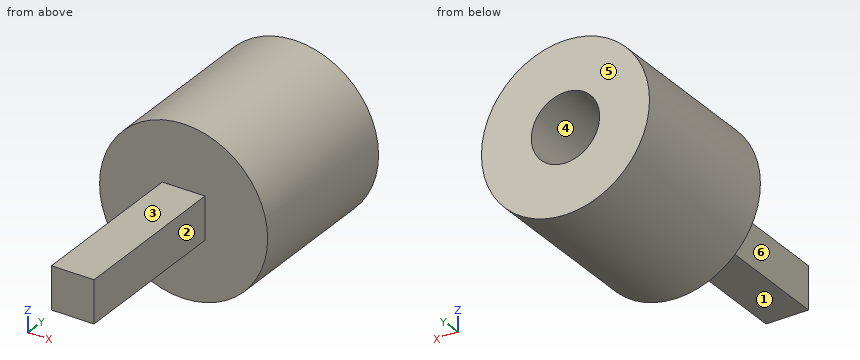
Autodesk Inventor part; units mm, degrees
ref_plane "YZ Plane" through (0, 0, 0) normal (1, 0, 0) x (0, 1, 0)
ref_plane "XZ Plane" through (0, 0, 0) normal (0, 1, 0) x (-1, 0, 0)
ref_plane "XY Plane" through (0, 0, 0) normal (0, 0, 1) x (1, 0, 0)
sketch "草圖1" plane through (0, 0, 0) normal (0, 1, 0) x (-1, 0, 0)
  circle A0 centre (0, 0) radius 7.5
  dimension "d0" = 15
extrude "擠出1" add sketch "草圖1" along normal blind 15
sketch "草圖2" plane through (0, 15, 0) normal (0, 1, 0) x (1, 0, 0)
  circle A0 centre (0, 0) radius 3.05
  dimension "d3" = 6.1
extrude "擠出2" cut sketch "草圖2" against normal blind 12
sketch "草圖3" plane through (0, 0, 0) normal (0, -1, 0) x (1, 0, 0)
  line L0 (1.9, 1.9) -> (-1.9, 1.9)
  line L1 (-1.9, 1.9) -> (-1.9, -1.9)
  line L2 (-1.9, -1.9) -> (1.9, -1.9)
  line L3 (1.9, -1.9) -> (1.9, 1.9)
  circle A0 centre (0, 0) radius 3.05
  line L4 (1.9, 1.9) -> (-1.9, -1.9) construction
  line L5 (-1.9, 1.9) -> (1.9, -1.9) construction
  dimension "d6" = 3.8
  dimension "d7" = 3.8
extrude "擠出3" add sketch "草圖3" along normal blind 15 contours L3 L2 L1 L0
properties part number "transfer"
The model under review builds one solid part; all positions refer to its coordinate system, in mm. Face numbers are marked on the shaded views. A direction names the side the tool comes from. Round coordinates to 2 decimals unless told otherwise and drop trailing zeros. Write each loop counter-clockwise with the first axis right and the second up, starting at its lowest first coordinate (ties: lowest second). Pieces come first, ordered by that corner, then holes. Notation, with made-up numbers: (73, 25) -> (95, 25) arc R11 cw to (95, 29) -> close; hole circle Ø11 at (22.5, 53.25). An arc over 180 degrees is marked (long way). Use CSV: the item, a comma, the result in double quotes.
Q1. To check wall thickness, follow probe 1 along Z at (x, y) = (0, 9); probe 2 along Y at (x, z) = (-3.75, -4.25); probe 3 along Z at (x, y) = (0.25, -5.5). State the ranges of each line that lie inside material, in increasing order. Write a range as [from, to].
Checks:
probe 1,"[-7.5, -3.05], [3.05, 7.5]"
probe 2,"[0, 15]"
probe 3,"[-1.9, 1.9]"
Q2. Consider section D-D (y = 10.25). Give the boundary of the cut face in (x, z).
Checks:
outline,"circle Ø15 at (0, 0); hole circle Ø6.1 at (0, 0)"
Q3. Mouldability with a two-part tool opening along X and no side actions: class the marked faces 4, 5 and 6 as released by +X, released by -X, zero draft, split by the parting line, or undercut.
Checks:
face 4,"undercut"
face 5,"zero draft"
face 6,"released by -X"
Q4. Consider section C-C (y = -11.5). Give the boundary of the cut face in (x, z).
Checks:
outline,"(-1.9, -1.9) -> (1.9, -1.9) -> (1.9, 1.9) -> (-1.9, 1.9) -> close"
Q5. Consider section A-A (x = 0). Give the boundary of the cut face in (y, z).
Checks:
outline,"(-15, -1.9) -> (0, -1.9) -> (0, -7.5) -> (15, -7.5) -> (15, -3.05) -> (3, -3.05) -> (3, 3.05) -> (15, 3.05) -> (15, 7.5) -> (0, 7.5) -> (0, 1.9) -> (-15, 1.9) -> close"
Q6. Consider section B-B (z = 0). Give the boundary of the cut face in (x, y), then the cut area to 3 significant figures.
Checks:
outline,"(-7.5, 0) -> (-1.9, 0) -> (-1.9, -15) -> (1.9, -15) -> (1.9, 0) -> (7.5, 0) -> (7.5, 15) -> (3.05, 15) -> (3.05, 3) -> (-3.05, 3) -> (-3.05, 15) -> (-7.5, 15) -> close"
area,"209 mm²"
Q7. For pin 1 Ø1.1 at (y, z) = (-10, -0.5) entering from -X; pin 2 Ø1.8 at (x, z) = (-0.5, -1) entering from +Y; pin 3 Ø6 at (x, y) = (-4, -10.5) entering from -Z, all flat-tipped, find the tip position at first contact; note any pin that passes through.
Checks:
pin 1,"x = -1.9"
pin 2,"y = 3"
pin 3,"z = -1.9"
Q8. For the marked faces 1, 2 and 3, list the 3-axis set-ups (+Z, -Z, +X, -X, +Y, -Y) from which the entire face can be reached by the end or side of a thin tool; tool diameter is ignored.
Checks:
face 1,"-Z, +X, -X, -Y"
face 2,"+Z, -Z, +X, -Y"
face 3,"+Z, +X, -X, -Y"
